Could you check a few things on this drawing? It's one solid part, dimensions in mm from its lowest x, y, z. Coordinates: 2 decimals unless noted, no trailing zeros. Write each loop counter-clockwise with the first axis right and the second up, starting at its lowest first coordinate (ties: lowest second). Pieces come first, ordered by that corner, then holes. Notation, with made-up numbers: (-9, 29) - (4, 29) arc R23 cw to (4, 68) - close; hole circle Ø2 at (34.5, 80.5). An arc over 180 degrees is marked (long way). Write item = value, one per line. Start each with the question number.
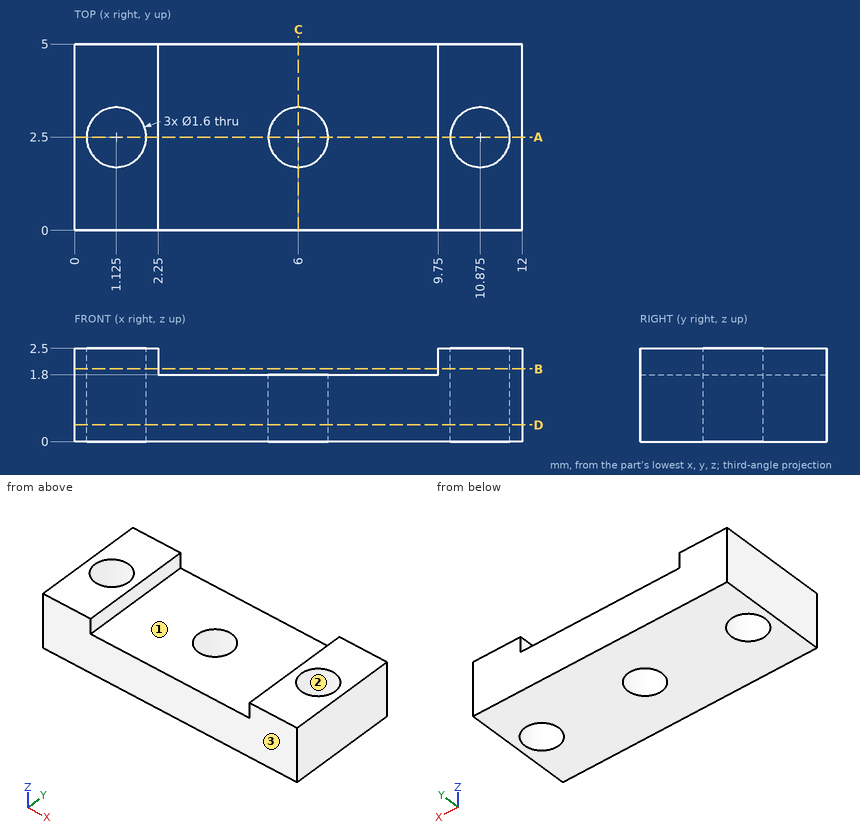
1) Suppose I cut it at D-D on z = 0.45. Please give me the cut outline in (x, y) (3 decimals), plus the area to 3 significant figures.
2) Suppose I cut it at A-A on y = 2.5. Please give me the cut outline in (x, z) (3 decimals).
3) For P1, Ø1.4, axis at x = 6, y = 2.5, coming from the -Z side, with a flat end and sliding along its axis, tell me the tip position at first contact or that it passes through.
4) If I drill on probe 1 along X at (y, z) = (2.8, 1); probe 2 along Z at (x, y) = (8.5, 0.45); probe 3 along X at (y, z) = (2.6, 1.4), over which ranges is the centre line in solid material (lowest first)? Write a range as [from, to].
5) Suppose I cut it at B-B on z = 1.95. Please give me the cut outline in (x, y) (3 decimals).
6) Suppose I cut it at C-C on x = 6. Please give me the cut outline in (y, z), plus the area to 3 significant figures.
7) Thinking about a two-plate mould opening in Y: for the marked faces 1, 2 and 3, which applies, +Y half, -Y half, draft (parallel to the pull), parting line (faces both ways), or undercut?
Reply:
q1.outline = (0, 0) - (12, 0) - (12, 5) - (0, 5) - close; hole circle Ø1.6 at (1.125, 2.5); hole circle Ø1.6 at (6, 2.5); hole circle Ø1.6 at (10.875, 2.5)
q1.area = 54.0 mm^2
q2.outline = (0, 0) - (0.325, 0) - (0.325, 2.5) - (0, 2.5) - close; (1.925, 0) - (5.2, 0) - (5.2, 1.8) - (2.25, 1.8) - (2.25, 2.5) - (1.925, 2.5) - close; (6.8, 0) - (10.075, 0) - (10.075, 2.5) - (9.75, 2.5) - (9.75, 1.8) - (6.8, 1.8) - close; (11.675, 0) - (12, 0) - (12, 2.5) - (11.675, 2.5) - close
q3.P1 = through
q4.probe_1 = [0, 0.38], [1.87, 5.26], [6.74, 10.13], [11.62, 12]
q4.probe_2 = [0, 1.8]
q4.probe_3 = [0, 0.33], [1.92, 5.21], [6.79, 10.08], [11.67, 12]
q5.outline = (0, 0) - (2.25, 0) - (2.25, 5) - (0, 5) - close; (9.75, 0) - (12, 0) - (12, 5) - (9.75, 5) - close; hole circle Ø1.6 at (1.125, 2.5); hole circle Ø1.6 at (10.875, 2.5)
q6.outline = (0, 0) - (1.7, 0) - (1.7, 1.8) - (0, 1.8) - close; (3.3, 0) - (5, 0) - (5, 1.8) - (3.3, 1.8) - close
q6.area = 6.12 mm^2
q7.face_1 = draft
q7.face_2 = undercut
q7.face_3 = -Y half
